Autodesk Inventor part; units mm, degrees
ref_plane "YZ Plane" through (0, 0, 0) normal (1, 0, 0) x (0, 1, 0)
ref_plane "XZ Plane" through (0, 0, 0) normal (0, 1, 0) x (-1, 0, 0)
ref_plane "XY Plane" through (0, 0, 0) normal (0, 0, 1) x (1, 0, 0)
sketch "Sketch1" plane through (0, 0, 0) normal (0, 1, 0) x (-1, 0, 0)
  arc A0 (0, -0.5) -> (0, 0.5) centre (0, 0) ccw
  arc A1 (0, -1.5) -> (0, 1.5) centre (0, 0) ccw
  line L0 (-13.5, -0.5) -> (0, -0.5)
  line L1 (-13.5, 0.5) -> (0, 0.5)
  line L2 (-13.5, -1.5) -> (0, -1.5)
  line L3 (-13.5, 1.5) -> (0, 1.5)
  line L4 (-13.5, -0.5) -> (-13.5, -1.5)
  line L5 (-13.5, 0.5) -> (-13.5, 1.5)
extrude "Extrusion1" add sketch "Sketch1" along normal mid plane 371.8
fillet "Fillet1" radius 1 4 edges at (13.5, 185.9, 1) (13.5, -185.9, 1) (13.5, 185.9, -1) (13.5, -185.9, -1)
properties part number "Binder"
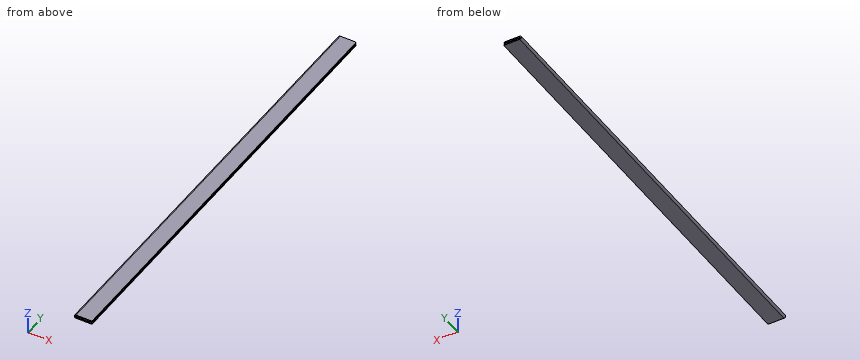
The listing builds one solid part. Answer for the finished solid, in the listing's coordinates (mm). Coordinates: 2 decimals unless noted, no trailing zeros. Write each loop counter-clockwise with the first axis right and the second up, starting at its lowest first coordinate (ties: lowest second). Pieces come first, ordered by that corner, then holes. Notation, with made-up numbers: M -37,41.25 L -31,41.25 A25 ccw -31,78.25 Z; hole C 67.25,-5 d8. An arc over 180 degrees is marked long. Use one line per item in the form item = value.
Item 1: Find the intervals of material crossed by probe 1 along Z at (x, y) = (7.75, 128.5); probe 2 along X at (y, z) = (-78, 0); probe 3 along X at (y, z) = (99.5, -0.7), in increasing order.
Model answer:
probe_1 = -1.5 to -0.5, 0.5 to 1.5
probe_2 = -1.5 to -0.5
probe_3 = -1.33 to 13.5
Item 2: Find section B-B, the plane y = 118.5. Give the vertices of the cut face in (x, z), plus the area to 3 significant figures.
Model answer:
outline = M 0,-1.5 L 13.5,-1.5 L 13.5,-0.5 L 0,-0.5 A0.5 cw 0,0.5 L 13.5,0.5 L 13.5,1.5 L 0,1.5 A1.5 ccw Z
area = 30.1 mm2
Item 3: Find section A-A, the plane x = 8.5. Give the vertices of the cut face in (y, z).
Model answer:
outline = M -185.9,-1.5 L 185.9,-1.5 L 185.9,-0.5 L -185.9,-0.5 Z; M -185.9,0.5 L 185.9,0.5 L 185.9,1.5 L -185.9,1.5 Z
Item 4: Find section C-C, the plane z = 0. Give the vertices of the cut face in (x, y).
Model answer:
outline = M -1.5,-185.9 L -0.5,-185.9 L -0.5,185.9 L -1.5,185.9 Z
